```python
from build123d import *

# Parameters (mm, degrees)
F0_W     = 183.51976946
F0_H     = 159.9090248346
F1_DEPTH = 127
F3_DEPTH = 159.9100248346
F5_DEPTH = 159.9100248346
F6_W     = 20.3265432715
F6_H     = 38.354692515
F7_DEPTH = 183.52076946


with BuildPart() as f1:
    # F0 (on Front) → F1 (new body)
    with BuildSketch(Plane.XZ):
        with Locations((33.8062848896, -26.8303751945)):
            Rectangle(F0_W, F0_H)
    extrude(amount=F1_DEPTH)

    # F2 (on face) → F3 (cut, through all)
    with BuildSketch(Plane(origin=(0, 0, -106.7848876119), x_dir=(1, 0, 0), z_dir=(0, 0, -1))):
        Polygon((61.1603185534, 201.0327279568), (125.5661696196, 0), (249.7815191746, 14.9288764223), (305.6204319, 25.561010465), align=None)
    extrude(amount=-F3_DEPTH, mode=Mode.SUBTRACT)

    # F4 (on face) → F5 (cut, through all)
    with BuildSketch(Plane.XY.offset(53.1241372228)):
        Polygon((127.3305118084, 0), (125.5661696196, 0), (32.5038395822, -127), (137.3508572578, -127), (149.5707929134, 0), align=None)
    extrude(amount=-F5_DEPTH, mode=Mode.SUBTRACT)

    # F6 (on face) → F7 (cut, through all)
    with BuildSketch(Plane(origin=(-57.9535998404, 0, 0), x_dir=(0, -1, 0), z_dir=(-1, 0, 0))):
        with Locations((116.8367283642, -24.4502548594)):
            Rectangle(F6_W, F6_H)
    extrude(amount=-F7_DEPTH, mode=Mode.SUBTRACT)


solid = f1.part
```
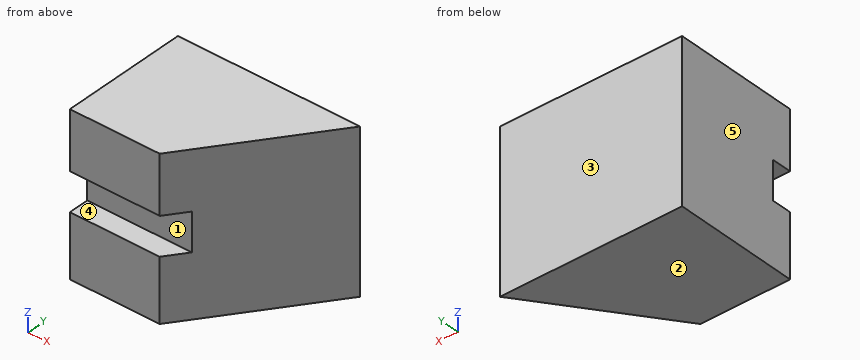
Verification items for the finished model (mm, model axes). Face numbers are marked on the shaded views. A direction names the side the tool comes from. Round coordinates to 2 decimals unless told otherwise and drop trailing zeros. Order: outer loops, then holes, each group sorted by start corner. A loop starts at its lowest first (then second) coordinate and runs counter-clockwise, first axis right, second up.
1) Material ranges on line 1 (Z direction, x = -18, y = -117); line 2 (Y direction, x = -31.5, z = -21.5); line 3 (Y direction, x = 114.5, z = -74), recorded low to high.
Geometry says:
line 1: z = -106.78 to -43.63, -5.27 to 53.12
line 2: y = -106.67 to 0
line 3: y = -15.1 to 0
2) Draft check along Z on the marked faces 1, 2 and 3. Enter one of: +Z half, -Z half, draft (parallel to the pull), parting line (faces both ways), or undercut.
Geometry says:
face 1: undercut
face 2: -Z half
face 3: draft
3) Depth check by flat-ended pin: pin 1 (8 mm diameter, centred on x = 54.5, z = -56.5, fed in from -Y); pin 2 (6 mm diameter, centred on y = -107, z = -59.5, fed in from +X); pin 3 (5 mm diameter, centred on y = -55.5, z = -69.5, fed in from +X). Enter the tip coordinate at first touch or a pass-through.
Geometry says:
pin 1: stops at y = -102.44
pin 2: stops at x = 49.36
pin 3: stops at x = 86.73
4) Cross-section at B-B, the plane z = 32.5. Record the cut outline in (x, y).
Geometry says:
outline: (-57.95, -127) - (32.5, -127) - (125.57, 0) - (-57.95, 0) - close
5) Tool access check on the marked faces 4 and 5. Record the directions out of +Z, -Z, +X, -X, +Y, -Y that give a thin tool (end or side, any length) a straight path to the whole face; none if there is none.
Geometry says:
face 4: +X, -X, -Y
face 5: +Z, -Z, -X, +Y, -Y
6) Cross-section at C-C, the plane y = -50. Record the cut outline in (x, z), plus the area to 3 significant figures.
Geometry says:
outline: (-57.95, -106.78) - (88.93, -106.78) - (88.93, 53.12) - (-57.95, 53.12) - close
area: 23,500 mm2
7) Cross-section at A-A, the plane x = 15.5. Record the cut outline in (y, z).
Geometry says:
outline: (-127, -106.78) - (0, -106.78) - (0, 53.12) - (-127, 53.12) - (-127, -5.27) - (-106.67, -5.27) - (-106.67, -43.63) - (-127, -43.63) - close
8) Cross-section at D-D, the plane x = 41.5. Record the cut outline in (y, z).
Geometry says:
outline: (-114.72, -106.78) - (0, -106.78) - (0, 53.12) - (-114.72, 53.12) - (-114.72, -5.27) - (-106.67, -5.27) - (-106.67, -43.63) - (-114.72, -43.63) - close
